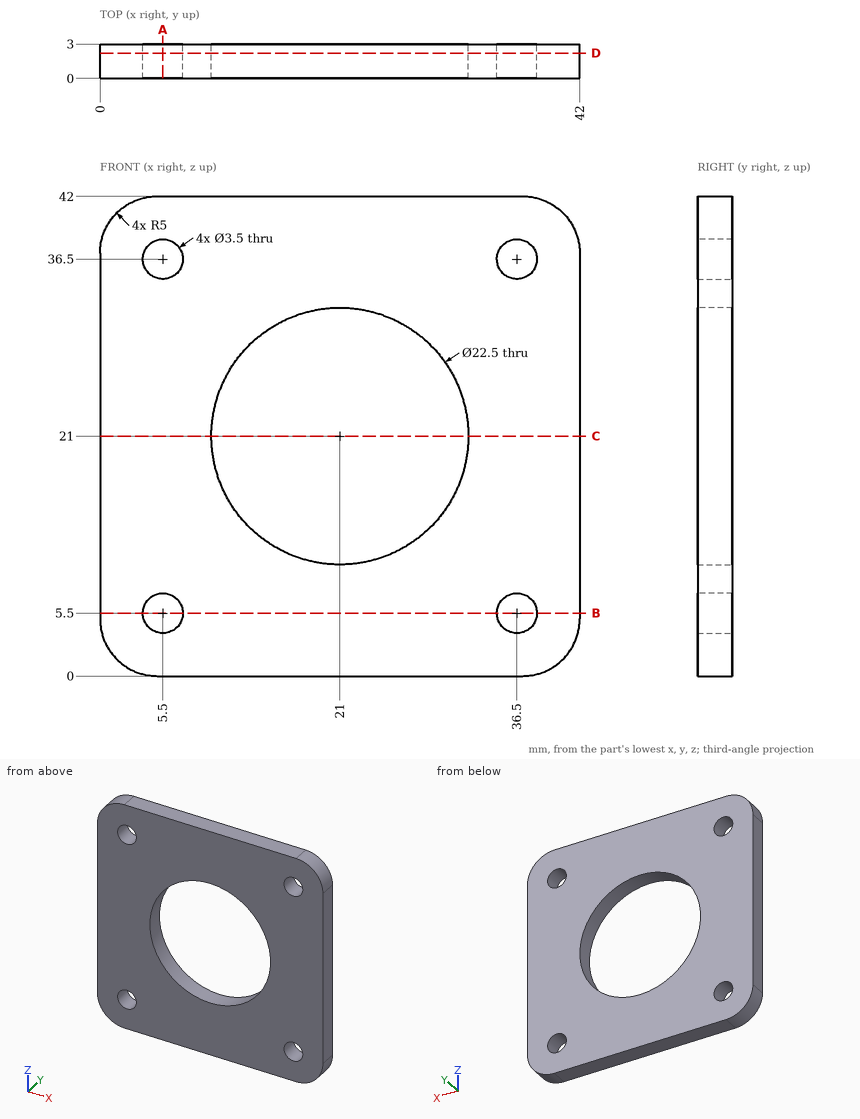
Can you work these out from the drawing? Everything is in mm from the part's minimum corner. Give positions to 0.01 mm unless a question says otherwise; leave off trailing zeros. Write each loop counter-clockwise with the first axis right and the second up, starting at its lowest first coordinate (ties: lowest second). Pieces come first, ordered by that corner, then holes. Notation, with made-up numbers: M -20.75,32 L 6.25,32 A18 ccw 6.25,65 Z; hole C 11,-20 d11. An arc over 180 degrees is marked long. Answer in a Markdown table with one row per item. Add a question column.
Item 1: Imagine slicing it at D-D, the plane y = 2.2. Write out the boundary of the cut face in (x, z).
Item 2: Imagine slicing it at B-B, the plane z = 5.5. Write out the boundary of the cut face in (x, y).
Item 3: For pin 1 Ø2 at (x, z) = (36.5, 36.5) entering from -Y, with a flat end and sliding along its axis, tell me the tip position at first contact or that it passes through.
Item 4: Please list where these lines run through material, in increasing order: L1, parallel to X at y = 1.15, z = 5.5; L2, parallel to Z at x = 21.5, y = 2.7; L3, parallel to X at y = 1.05, z = 7.
Item 5: Imagine slicing it at C-C, the plane z = 21. Write out the boundary of the cut face in (x, y).
Item 6: Imagine slicing it at A-A, the plane x = 5.5. Write out the boundary of the cut face in (y, z), plus the area to 3 significant figures.
Evaluation:
| question | item | result |
|---|---|---|
| 1 | outline | M 0,5 A5 ccw 5,0 L 37,0 A5 ccw 42,5 L 42,37 A5 ccw 37,42 L 5,42 A5 ccw 0,37 Z; hole C 5.5,5.5 d3.5; hole C 5.5,36.5 d3.5; hole C 21,21 d22.5; hole C 36.5,5.5 d3.5; hole C 36.5,36.5 d3.5 |
| 2 | outline | M 0,0 L 3.75,0 L 3.75,3 L 0,3 Z; M 7.25,0 L 34.75,0 L 34.75,3 L 7.25,3 Z; M 38.25,0 L 42,0 L 42,3 L 38.25,3 Z |
| 3 | pin 1 | passes through |
| 4 | L1 | x = 0 to 3.75, 7.25 to 34.75, 38.25 to 42 |
| 4 | L2 | z = 0 to 9.76, 32.24 to 42 |
| 4 | L3 | x = 0 to 4.6, 6.4 to 35.6, 37.4 to 42 |
| 5 | outline | M 0,0 L 9.75,0 L 9.75,3 L 0,3 Z; M 32.25,0 L 42,0 L 42,3 L 32.25,3 Z |
| 6 | outline | M 0,0 L 3,0 L 3,3.75 L 0,3.75 Z; M 0,7.25 L 3,7.25 L 3,34.75 L 0,34.75 Z; M 0,38.25 L 3,38.25 L 3,42 L 0,42 Z |
| 6 | area | 105 mm² |
